Read the model definition and answer for the solid it produces. Units are mm, in the model's axes. Face numbers are marked on the shaded views. A direction names the side the tool comes from. Round coordinates to 2 decimals unless told otherwise and drop trailing zeros. Write each loop counter-clockwise with the first axis right and the second up, starting at its lowest first coordinate (ties: lowest second). Pieces come first, ordered by that corner, then holes.
from build123d import *

# Parameters (mm, degrees)
ESQUISSE1_R                  = 10.4775
BOSS_EXTRU_1_DEPTH           = 7.62
ESQUISSE3_R                  = 4.1275
ENL_V_MAT_EXTRU_1_DEPTH      = 2.286
ESQUISSE4_R                  = 2.413
ENL_V_MAT_EXTRU_2_DEPTH      = 2.286
BOSS_EXTRU_2_DEPTH           = 19.05
ESQUISSE6_R                  = 1.27
ENL_V_MAT_EXTRU_3_DEPTH      = 1
ENL_V_MAT_EXTRU_3_DEPTH_BACK = 27.67
ESQUISSE7_R                  = 1.651
ENL_V_MAT_EXTRU_4_DEPTH      = 4.318
CHANFREIN1_SIZE              = 0.3175
CONG_1_R                     = 0.762


with BuildPart() as part:
    # Esquisse1 → Boss.-Extru.1 (new body)
    with BuildSketch(Plane.XY):
        with Locations((0, 12)):
            Circle(ESQUISSE1_R)
    extrude(amount=BOSS_EXTRU_1_DEPTH)

    # Esquisse3 → Enlèv. mat.-Extru.1 (cut)
    with BuildSketch(Plane(origin=(0, 0, 0), x_dir=(-1, 0, 0), z_dir=(0, 0, -1))):
        with Locations((0, 12)):
            Circle(ESQUISSE3_R)
    extrude(amount=-ENL_V_MAT_EXTRU_1_DEPTH, mode=Mode.SUBTRACT)

    # Esquisse4 → Enlèv. mat.-Extru.2 (cut)
    with BuildSketch(Plane(origin=(0, 0, 2.286), x_dir=(-1, 0, 0), z_dir=(0, 0, -1))):
        with Locations((0, 12)):
            Circle(ESQUISSE4_R)
    extrude(amount=-ENL_V_MAT_EXTRU_2_DEPTH, mode=Mode.SUBTRACT)

    # Esquisse5 → Boss.-Extru.2 (add)
    with BuildSketch(Plane.XY.offset(7.62)):
        with BuildLine():
            Line((-1.905, 14.54), (1.905, 14.54))
            ThreePointArc((1.905, 14.54), (0, 8.825), (-1.905, 14.54))
        make_face()
    extrude(amount=BOSS_EXTRU_2_DEPTH)

    # Esquisse6 → Enlèv. mat.-Extru.3 (cut, two sides)
    with BuildSketch(Plane(origin=(0, 0, 0), x_dir=(-1, 0, 0), z_dir=(0, 0, -1))) as enl_v_mat_extru_3_sk:
        with Locations((-5.656854249, 17.656854249)):
            Circle(ESQUISSE6_R)
        with Locations((5.656854249, 17.656854249)):
            Circle(ESQUISSE6_R)
        with Locations((5.656854249, 6.343145751)):
            Circle(ESQUISSE6_R)
        with Locations((-5.656854249, 6.343145751)):
            Circle(ESQUISSE6_R)
    extrude(amount=ENL_V_MAT_EXTRU_3_DEPTH, mode=Mode.SUBTRACT)
    extrude(enl_v_mat_extru_3_sk.sketch, amount=-ENL_V_MAT_EXTRU_3_DEPTH_BACK, mode=Mode.SUBTRACT)

    # Esquisse7 → Enlèv. mat.-Extru.4 (cut)
    with BuildSketch(Plane.XY.offset(7.62)):
        with Locations((-5.656854249, 17.656854249)):
            Circle(ESQUISSE7_R)
        with Locations((5.656854249, 17.656854249)):
            Circle(ESQUISSE7_R)
        with Locations((5.656854249, 6.343145751)):
            Circle(ESQUISSE7_R)
        with Locations((-5.656854249, 6.343145751)):
            Circle(ESQUISSE7_R)
    extrude(amount=-ENL_V_MAT_EXTRU_4_DEPTH, mode=Mode.SUBTRACT)

    # Chanfrein1
    chanfrein1_edges = [part.edges().sort_by_distance(p)[0] for p in [
        (-10.4775, 12, 7.62),
    ]]
    chamfer(chanfrein1_edges, length=CHANFREIN1_SIZE)

    # Congé1
    cong_1_edges = [part.edges().sort_by_distance(p)[0] for p in [
        (0, 8.825, 7.62),
        (0, 14.54, 7.62),
    ]]
    fillet(cong_1_edges, radius=CONG_1_R)


solid = part.part
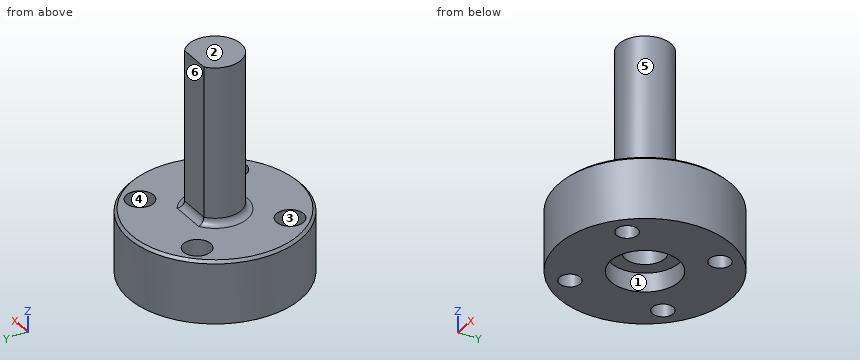
Q1. Section C-C (z = 8.75) is taken. Determine the outline of the cut face in (x, y) (3 decimals).
Verdict:
outline: (-1.905, 14.54) arc R3.175 ccw (long way) to (1.905, 14.54) - close
Q2. Flat-ended cylindrical pins translate along their axes: pin 1 Ø10 at (x, y) = (0, 7.5) entering from -Z; pin 2 Ø1.7 at (x, y) = (5, 18) entering from +Z; pin 3 Ø1.5 at (x, z) = (4.5, 5.5) entering from +Y; pin 4 Ø1.4 at (x, y) = (-0.5, 11) entering from -Z. Find the tip coordinate at first contact, or state that the pin passes through.
Verdict:
pin 1: stops at z = 0
pin 2: stops at z = 3.3
pin 3: stops at y = 21.78
pin 4: stops at z = 4.57
Q3. Section B-B (y = 12) is taken. Determine the outline of the cut face in (x, z) (1 decimal).
Verdict:
outline: (-10.5, 0) - (-4.1, 0) - (-4.1, 2.3) - (-2.4, 2.3) - (-2.4, 4.6) - (2.4, 4.6) - (2.4, 2.3) - (4.1, 2.3) - (4.1, 0) - (10.5, 0) - (10.5, 7.3) - (10.2, 7.6) - (3.9, 7.6) arc R0.8 cw to (3.2, 8.4) - (3.2, 26.7) - (-3.2, 26.7) - (-3.2, 8.4) arc R0.8 cw to (-3.9, 7.6) - (-10.2, 7.6) - (-10.5, 7.3) - close
Q4. Which of the six approach directions +Z, -Z, +X, -X, +Y, -Y give full straight-line access (tool end or side, diameter ignored) to the marked faces 1, 2 and 3?
Verdict:
face 1: -Z
face 2: +Z, +X, -X, +Y, -Y
face 3: +Z
Q5. Determine the mould class of the marked faces 4, 5 and 6 for opening direction Y: pulls with the +Y half, pulls with the -Y half, needs draft (parallel to the pull), parting line crosses it, or undercut.
Verdict:
face 4: undercut
face 5: parting line crosses it
face 6: pulls with the +Y half
Q6. Section D-D (y = 6) is taken. State how many separate pieces and enclosed holes the cut face has, then the cut area to 3 significant figures.
Verdict:
separate pieces: 3
enclosed holes: 0
area: 86.7 mm2
Q7. Straight lines are drawn through the part: probe 1 along Y at (x, z) = (0, 0.7); probe 2 along X at (y, z) = (17.75, 7.5); probe 3 along X at (y, z) = (18.25, 7.5). For each, find the intervals that lie inside material, in ascending order.
Verdict:
probe 1: y = 1.52 to 7.87, 16.13 to 22.48
probe 2: x = -8.52 to -7.31, -4.01 to 4.01, 7.31 to 8.52
probe 3: x = -8.16 to -7.2, -4.12 to 4.12, 7.2 to 8.16
Q8. Section A-A (x = 0) is taken. Determine the outline of the cut face in (y, z) (1 decimal), then the cut area to 3 significant figures.
Verdict:
outline: (1.5, 0) - (7.9, 0) - (7.9, 2.3) - (9.6, 2.3) - (9.6, 4.6) - (14.4, 4.6) - (14.4, 2.3) - (16.1, 2.3) - (16.1, 0) - (22.5, 0) - (22.5, 7.3) - (22.2, 7.6) - (15.3, 7.6) arc R0.8 cw to (14.5, 8.4) - (14.5, 26.7) - (8.8, 26.7) - (8.8, 8.4) arc R0.8 cw to (8.1, 7.6) - (1.8, 7.6) - (1.5, 7.3) - close
area: 239 mm2
